from build123d import *

# Parameters (mm, degrees)
SKETCH1_W           = 40.7
SKETCH1_H           = 19.9
BOSS_EXTRUDE1_DEPTH = 41.1
SKETCH2_W           = 54.1
SKETCH2_H           = 4.5
BOSS_EXTRUDE2_DEPTH = 19.9
CUT_EXTRUDE1_REACH  = 34.2
SKETCH3_R           = 2.25
SKETCH4_R           = 3
BOSS_EXTRUDE3_DEPTH = 3.7
SKETCH6_W           = 4.5
SKETCH6_H           = 6.7
BOSS_EXTRUDE4_DEPTH = 5.5


with BuildPart() as part:
    # Sketch1 → Boss-Extrude1 (new body)
    with BuildSketch(Plane.XY):
        Rectangle(SKETCH1_W, SKETCH1_H)
    extrude(amount=BOSS_EXTRUDE1_DEPTH)

    # Sketch2 → Boss-Extrude2 (add)
    with BuildSketch(Plane.XZ.offset(9.95)):
        with Locations((0, 29.95)):
            Rectangle(SKETCH2_W, SKETCH2_H)
    extrude(amount=-BOSS_EXTRUDE2_DEPTH)

    # Sketch3 → Cut-Extrude1 (cut, up to next)
    with BuildSketch(Plane.XY.offset(32.2), mode=Mode.PRIVATE) as cut_extrude1_sk1:
        with Locations((-25.25, 4.649810013)):
            Circle(SKETCH3_R)
    cut_extrude1_tool1 = extrude(cut_extrude1_sk1.sketch, amount=-CUT_EXTRUDE1_REACH, mode=Mode.PRIVATE) & part.part
    add(cut_extrude1_tool1.solids().sort_by_distance((-25.25, 4.64981, 32.2))[0], mode=Mode.SUBTRACT)
    # Sketch3 → Cut-Extrude1 (cut, up to next)
    with BuildSketch(Plane.XY.offset(32.2), mode=Mode.PRIVATE) as cut_extrude1_sk2:
        with Locations((-25.25, -5.350189987)):
            Circle(SKETCH3_R)
    cut_extrude1_tool2 = extrude(cut_extrude1_sk2.sketch, amount=-CUT_EXTRUDE1_REACH, mode=Mode.PRIVATE) & part.part
    add(cut_extrude1_tool2.solids().sort_by_distance((-25.25, -5.35019, 32.2))[0], mode=Mode.SUBTRACT)
    # Sketch3 → Cut-Extrude1 (cut, up to next)
    with BuildSketch(Plane.XY.offset(32.2), mode=Mode.PRIVATE) as cut_extrude1_sk3:
        with Locations((25.25, 4.649810013)):
            Circle(SKETCH3_R)
    cut_extrude1_tool3 = extrude(cut_extrude1_sk3.sketch, amount=-CUT_EXTRUDE1_REACH, mode=Mode.PRIVATE) & part.part
    add(cut_extrude1_tool3.solids().sort_by_distance((25.25, 4.64981, 32.2))[0], mode=Mode.SUBTRACT)
    # Sketch3 → Cut-Extrude1 (cut, up to next)
    with BuildSketch(Plane.XY.offset(32.2), mode=Mode.PRIVATE) as cut_extrude1_sk4:
        with Locations((25.25, -5.350189987)):
            Circle(SKETCH3_R)
    cut_extrude1_tool4 = extrude(cut_extrude1_sk4.sketch, amount=-CUT_EXTRUDE1_REACH, mode=Mode.PRIVATE) & part.part
    add(cut_extrude1_tool4.solids().sort_by_distance((25.25, -5.35019, 32.2))[0], mode=Mode.SUBTRACT)

    # Sketch4 → Boss-Extrude3 (add)
    with BuildSketch(Plane.XY.offset(41.1)):
        with Locations((-10.4, 0)):
            Circle(SKETCH4_R)
    extrude(amount=BOSS_EXTRUDE3_DEPTH)

    # Sketch6 → Boss-Extrude4 (add)
    with BuildSketch(Plane.ZY.offset(20.35)):
        with Locations((5.75, 0)):
            Rectangle(SKETCH6_W, SKETCH6_H)
    extrude(amount=BOSS_EXTRUDE4_DEPTH)


solid = part.part
Source: CAD feature listing. Evaluate the final solid. Frame: model axes, mm. A direction names the side the tool comes from. Give positions to 0.01 mm unless a question says otherwise; leave off trailing zeros. Write each loop counter-clockwise with the first axis right and the second up, starting at its lowest first coordinate (ties: lowest second). Pieces come first, ordered by that corner, then holes. Notation, with made-up numbers: M 66,-18.5 L 115,-18.5 A4 ccw 115,-13.5 Z; hole C -37,39 d4. An arc over 180 degrees is marked long. Return JSON: item names as keys, results as strings. Group by question number.
1) Set-up query: faces 1 (the face through (-23, 0, 32.2)), 2 (the face through (-23, 0, 8)), 3 (the face through (20.35, 0, 14)), 4 (the face through (-25.85, 0, 6)). Return all of +Z, -Z, +X, -X, +Y, -Y with unobstructed straight access to the full face (end or side cutting, diameter ignored); none if empty.
2) Cut plane A-A, the plane x = 25.25. Output: boundary loops of the cut face in (y, z), plus the area to 4 significant figures.
3) Cut plane D-D, the plane x = -10.4. Output: boundary loops of the cut face in (y, z).
4) Material intervals for line 1 along Y through (x, z) = (-25.25, 30.2); line 2 along X through (y, z) = (-3.75, 31); line 3 along Z through (x, y) = (6, 6), sorted ascending. Write a range as [from, to].
5) Pin query (flat end, axial travel): P1, Ø5, axis at x = -22.5, z = 5.5, coming from the +Y side; P2, Ø8, axis at y = -2, z = 23, coming from the +X side; P3, Ø3.5, axis at x = -24, y = 0.5, coming from the +Z side; P4, Ø3.5, axis at y = 1, z = 6.5, coming from the -X side. Return the tip coordinate at first contact, or that it passes through.
6) Cut plane B-B, the plane y = -8.25. Output: boundary loops of the cut face in (x, z), plus the area to 3 significant figures.
7) Cut plane C-C, the plane x = -25.25. Output: boundary loops of the cut face in (y, z).
8) Pull-direction query (X, two-part tool) for faces 5 (the face through (-27.05, 0, 30)), 6 (the face through (-13.4, 0.1, 42.9)), 7 (the face through (-23, 4.6, 30)); classes: pulls with the +X half, pulls with the -X half, needs draft (parallel to the pull), parting line crosses it, or undercut.
Recorded:
{
 "1": {"face 1": "+Z, -X, +Y, -Y", "face 2": "-X, +Y, -Y", "face 3": "-Z, +X, +Y, -Y", "face 4": "-Z, -X, +Y, -Y"},
 "2": {"outline": "M -9.95,27.7 L -7.6,27.7 L -7.6,32.2 L -9.95,32.2 Z; M -3.1,27.7 L 2.4,27.7 L 2.4,32.2 L -3.1,32.2 Z; M 6.9,27.7 L 9.95,27.7 L 9.95,32.2 L 6.9,32.2 Z", "area": "49.05 mm²"},
 "3": {"outline": "M -9.95,0 L 9.95,0 L 9.95,41.1 L 3,41.1 L 3,44.8 L -3,44.8 L -3,41.1 L -9.95,41.1 Z"},
 "4": {"line 1": "y = [-9.95, -7.6], [-3.1, 2.4], [6.9, 9.95]", "line 2": "x = [-27.05, -26.83], [-23.67, 23.67], [26.83, 27.05]", "line 3": "z = [0, 41.1]"},
 "5": {"P1": "stops at y = 9.95", "P2": "stops at x = 20.35", "P3": "stops at z = 32.2", "P4": "stops at x = -25.85"},
 "6": {"outline": "M -27.05,27.7 L -20.35,27.7 L -20.35,0 L 20.35,0 L 20.35,27.7 L 27.05,27.7 L 27.05,32.2 L 20.35,32.2 L 20.35,41.1 L -20.35,41.1 L -20.35,32.2 L -27.05,32.2 Z", "area": "1,730 mm²"},
 "7": {"outline": "M -9.95,27.7 L -7.6,27.7 L -7.6,32.2 L -9.95,32.2 Z; M -3.35,3.5 L 3.35,3.5 L 3.35,8 L -3.35,8 Z; M -3.1,27.7 L 2.4,27.7 L 2.4,32.2 L -3.1,32.2 Z; M 6.9,27.7 L 9.95,27.7 L 9.95,32.2 L 6.9,32.2 Z"},
 "8": {"face 5": "pulls with the -X half", "face 6": "parting line crosses it", "face 7": "undercut"}
}
